The model under review builds one solid part; all positions refer to its coordinate system, in mm. Face numbers are marked on the shaded views. A direction names the side the tool comes from. Give positions to 0.01 mm unless a question says otherwise; leave off trailing zeros. Loops run counter-clockwise (first coordinate to the right, second up) from the corner with the lowest first, then second, coordinate; pieces in that order, holes last. Notation, with made-up numbers: (30, 34) - (78, 34) arc R22 ccw to (78, 44) - close; hole circle Ø6 at (-21, 58.25). An arc over 180 degrees is marked (long way). Return JSON: item names as keys, results as strings. Group by question number.
from build123d import *

# Parameters (mm, degrees)
F1_DEPTH = 46.736
F3_DEPTH = 103.124


with BuildPart() as f1:
    # F0 (on Right) → F1 (new body)
    with BuildSketch(Plane.YZ):
        Polygon((-11.445979, 114.554122), (-19.315097, 34.645349), (-125.190452, 47.106925), (0, -18.487986), (13.276745, -80.830555), (43.63782, -33.176992), (158.097655, -106.101729), (78.691132, -18.487986), (122.328952, 26.189538), (32.907203, 30.837342), align=None)
    extrude(amount=-F1_DEPTH)

    # F2 (on face) → F3 (cut)
    with BuildSketch(Plane.YZ):
        Polygon((-14.845758, 27.206887), (-90.865381, 36.15443), (5.442825, -9.693216), (16.382012, -61.059497), (40.33051, -23.470866), (112.687898, -69.57126), (66.389852, -18.487986), (106.984551, 23.073913), (27.467924, 27.206887), (-8.213498, 94.555692), align=None)
    extrude(amount=-F3_DEPTH, mode=Mode.SUBTRACT)


solid = f1.part
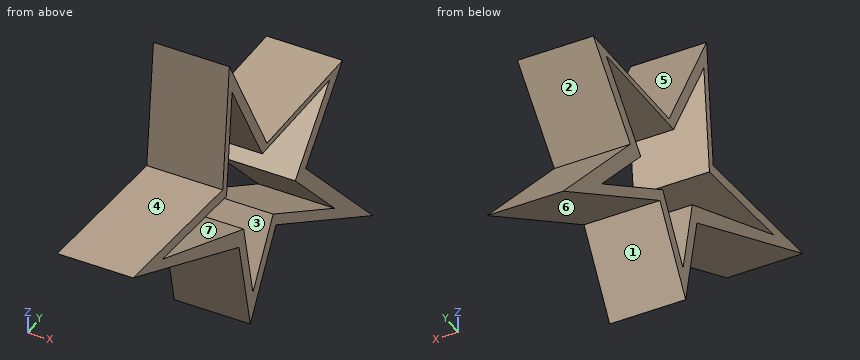
Item 1: Take a section at C-C (y = -46). State the section outline as (x, z) points, then the cut area to 3 significant figures.
Item 2: For P1, Ø3, axis at x = -10, y = 80, coming from the +Z side; P2, Ø8, axis at x = -6.5, z = -20, coming from the -Y side; P3, Ø2, axis at x = -35, z = 20.5, coming from the +Y side; P4, Ø12, axis at y = -38.5, z = -11, coming from the -X side, all flat-tipped, find the tip position at first contact; note any pin that passes through.
Item 3: Mouldability with a two-part tool opening along Z and no side actions: class the marked faces 5, 6 and 7 as +Z half, -Z half, draft (parallel to the pull), parting line (faces both ways), or undercut.
Item 4: Tool access review of the marked faces 1, 2, 3 and 4: name each direction out of +Z, -Z, +X, -X, +Y, -Y from which nothing blocks a thin tool from reaching the whole face with its end or side.
Item 5: Take a section at A-A (x = -18.5). State the section outline as (y, z) points.
Item 6: For L1, parallel to Z at x = -18.5, y = 99; L2, parallel to Y at x = -7, z = -30.5; L3, parallel to Y at x = -39.5, z = -26.5, list the stretches that pass through material, from the lowest coordinate up. Write a range as from..to.
Item 7: Take a section at B-B (z = -65). State the section outline as (x, y) points.
Item 8: Take a section at D-D (z = -6). State the section outline as (x, y) points, then the cut area to 3 significant figures.
Check sheet entries:
{
 "1": {"outline": "(-46.74, 5.61) - (0, 5.61) - (0, 14.8) - (-46.74, 14.8) - close; (-46.74, 30.87) - (0, 30.87) - (0, 37.79) - (-46.74, 37.79) - close", "area": "752 mm^2"},
 "2": {"P1": "stops at z = 28.47", "P2": "stops at y = -4.75", "P3": "stops at y = 117.75", "P4": "passes through"},
 "3": {"face 5": "+Z half", "face 6": "-Z half", "face 7": "undercut"},
 "4": {"face 1": "-Z, +X, -X", "face 2": "+X, -X, +Y", "face 3": "+X, -X", "face 4": "+Z, +X, -X"},
 "5": {"outline": "(-125.19, 47.11) - (0, -18.49) - (13.28, -80.83) - (43.64, -33.18) - (158.1, -106.1) - (78.69, -18.49) - (122.33, 26.19) - (32.91, 30.84) - (-11.45, 114.55) - (-19.32, 34.65) - close; hole (-90.87, 36.15) - (5.44, -9.69) - (16.38, -61.06) - (40.33, -23.47) - (112.69, -69.57) - (66.39, -18.49) - (106.98, 23.07) - (27.47, 27.21) - (-8.21, 94.56) - (-14.85, 27.21) - close"},
 "6": {"L1": "z = -68.45..-60.85, -54.47..-40.9, 2.3..14.9, 23.49..27.4", "L2": "y = 2.56..9.87, 35.85..51.36, 77.28..89.58", "L3": "y = 1.71..9.02, 38.4..45.08, 73.65..85.95"},
 "7": {"outline": "(-46.74, 9.91) - (0, 9.91) - (0, 23.36) - (-46.74, 23.36) - close; (-46.74, 93.59) - (0, 93.59) - (0, 105.51) - (-46.74, 105.51) - close; (-46.74, 108.54) - (0, 108.54) - (0, 120.85) - (-46.74, 120.85) - close"},
 "8": {"outline": "(-46.74, -23.83) - (0, -23.83) - (0, -2.32) - (-46.74, -2.32) - close; (-46.74, 78.59) - (0, 78.59) - (0, 90.89) - (-46.74, 90.89) - close", "area": "1,580 mm^2"}
}
